Read the model definition and answer for the solid it produces. Units are mm, in the model's axes. Coordinates: 2 decimals unless noted, no trailing zeros. Loops run counter-clockwise (first coordinate to the right, second up) from the corner with the lowest first, then second, coordinate; pieces in that order, holes last.
Q1. Section A-A (x = 3.25) is taken. Give the vertices of the cut face in (y, z), then the cut area to 3 significant figures.
Q2. The mould has two halves that part along Y. Classify faces 1 (the face through (5.344, -1.802, 5.723)), 2 (the face through (0, 3.3, 0.1)), 3 (the face through (5.8, -1.5, -2.6)): pulls with the +Y half, pulls with the -Y half, needs draft (parallel to the pull), parting line crosses it, or undercut.
Q3. Straight lines are drawn through the part: line 1 (Y direction, x = 6.75, z = 0); line 2 (Y direction, x = 6, z = -2.75); line 3 (Z direction, x = 7, y = -0.5). For each, find the intervals that lie inside material, in ascending order.
Q4. Section B-B (z = 0) is taken. Give the vertices of the cut face in (x, y), then the cut area to 3 significant figures.
Q5. Flat-ended cylindrical pins translate along their axes: P1, Ø1.5, axis at x = 6.5, y = -4, coming from the -Z side; P2, Ø1, axis at x = 5, z = 3.5, coming from the -Y side; P3, Ø1.5, axis at x = 3, y = 2.5, coming from the +Z side. Find the tip coordinate at first contact, or state that the pin passes through.
from build123d import *

# Parameters (mm, degrees)
HEX_2_DEPTH = 15.696938457


with BuildPart() as part:
    # BodySke → BaseBody (revolve)
    with BuildSketch(Plane.XY, mode=Mode.PRIVATE) as basebody_sk:
        Polygon((0, 0), (0, 5.036), (0.556565659, 6), (10, 6), (12, 4), (9.690598923, 0), align=None)
    revolve(basebody_sk.sketch.rotate(Axis((-12.7, 0, 0), (1, 0, 0)), 90), axis=Axis((-12.7, 0, 0), (1, 0, 0)))

    # Sketch2 → Hex 2 (cut, through all)
    with BuildSketch(Plane.ZY):
        Polygon((1.732050808, 3), (-1.732050808, 3), (-3.464101615, 0), (-1.732050808, -3), (1.732050808, -3), (3.464101615, 0), align=None)
    extrude(amount=-HEX_2_DEPTH, mode=Mode.SUBTRACT)


solid = part.part
Numbers:
1. outline: circle Ø12 at (0, 0); hole (-3, -1.73) - (0, -3.46) - (3, -1.73) - (3, 1.73) - (0, 3.46) - (-3, 1.73) - close
1. area: 81.9 mm2
2. face 1: parting line crosses it
2. face 2: needs draft
2. face 3: undercut
3. line 1: y = -6 to -3, 3 to 6
3. line 2: y = -5.33 to -1.24, 1.24 to 5.33
3. line 3: z = -5.98 to -3.18, 3.18 to 5.98
4. outline: (0, -5.04) - (0.56, -6) - (10, -6) - (12, -4) - (11.42, -3) - (0, -3) - close; (0, 3) - (11.42, 3) - (12, 4) - (10, 6) - (0.56, 6) - (0, 5.04) - close
4. area: 66.9 mm2
5. P1: stops at z = -5.04
5. P2: stops at y = -5.2
5. P3: stops at z = 5.74
